Build history of the part. All positions in model axes, mm. Round coordinates to 2 decimals unless told otherwise and drop trailing zeros. Loops run counter-clockwise (first coordinate to the right, second up) from the corner with the lowest first, then second, coordinate; pieces in that order, holes last. Notation, with made-up numbers: (-38.5, -32) - (-21.5, -32) arc R14 cw to (-21.5, -13) - close; hole circle Ø2 at (82.25, 66.25). An arc over 180 degrees is marked (long way). Put each result on its own line as item: value. Start each with the question number.
from build123d import *

# Parameters (mm, degrees)
F0_R      = 21.5
F1_DEPTH  = 8
F3_R      = 15
F1_FACE_R = 21.5
F6_D      = 6.8
F6_DEPTH  = 25
F6_TIP    = 2.0429261047
F7_R      = 2


with BuildPart() as f1:
    # F0 (on Top) → F1 (new body)
    with BuildSketch(Plane.XY):
        Circle(F0_R)
    extrude(amount=F1_DEPTH)

    # F3 (on offset) → F4 section 0
    with BuildSketch(Plane.XY.offset(43)):
        Circle(F3_R)
    # F1_face (on face) → F4 section 1
    with BuildSketch(Plane.XY.offset(8)):
        Circle(F1_FACE_R)
    loft()

    # F6
    with Locations(Plane(origin=(0, 0, 0), x_dir=(1, 0, 0), z_dir=(0, 0, -1))):
        with Locations((0, 0)):
            Hole(F6_D / 2, depth=F6_DEPTH)
            with Locations((0, 0, -(F6_DEPTH + F6_TIP / 2))):  # 118° drill point
                Cone(0, F6_D / 2, F6_TIP, mode=Mode.SUBTRACT)

    # F7
    f7_edges = [f1.edges().sort_by_distance(p)[0] for p in [
        (-15, 0, 43),
    ]]
    fillet(f7_edges, radius=F7_R)


solid = f1.part
Item 1: Slice it at A-A (z = 22). Give the cut face in (x, y).
Item 2: Drill centre lines: probe 1 along Y at (x, z) = (0, 7); probe 2 along Y at (x, z) = (0, 16); probe 3 along X at (y, z) = (-3, 4.5). Where is each one in solid material? Low to high. Write a range as [from, to].
Item 3: Two-plate mould, pull along X, no slides. Class faces 1 (the conical face through (-14.091, -10.805, 28.156)), 2 (the flat face through (4, 0, 0)), 3 (the cylindrical face through (0.74, 3.32, 12.67)): pulls with the +X half, pulls with the -X half, needs draft (parallel to the pull), parting line crosses it, or undercut.
Item 4: Slice it at B-B (z = 3.5). Give the cut face in (x, y).
Item 5: Drop flat-ended pins along their axis: pin 1 Ø1.5 at (x, z) = (7.5, 21) entering from +Y; pin 2 Ø10 at (x, z) = (8.5, 12.5) entering from +Y; pin 3 Ø10 at (y, z) = (3, 30.5) entering from -X. Give the stop position or say it passes through.
Computed values:
1. outline: circle Ø37.8 at (0, 0); hole circle Ø6.8 at (0, 0)
2. probe 1: y = [-21.5, -3.4], [3.4, 21.5]
2. probe 2: y = [-20.01, -3.4], [3.4, 20.01]
2. probe 3: x = [-21.29, -1.6], [1.6, 21.29]
3. face 1: parting line crosses it
3. face 2: needs draft
3. face 3: undercut
4. outline: circle Ø43 at (0, 0); hole circle Ø6.8 at (0, 0)
5. pin 1: stops at y = 17.89
5. pin 2: stops at y = 20.74
5. pin 3: stops at x = -18.15
